Geometry: see drawing. Coordinates: mm, zero at the bounding-box minimum. Give positions to 0.01 mm unless a question says otherwise; leave off trailing zeros. Answer as a JSON object with one key per item and string values. Group by question number.
1. Material intervals for L1, parallel to Y at x = 3.25, z = 4.5 (1 decimal); L2, parallel to Y at x = 2.25, z = 10.75 (1 decimal); L3, parallel to Y at x = 5.75, z = 6.5, sorted ascending. Write a range as [from, to].
2. Section query A-A (x = 4). Count the separate pieces of the cut face and the enclosed holes in it, plus the area to 3 significant figures.
3. Pin query (flat end, axial travel): P1, Ø2, axis at x = 3.18, y = 52.39, coming from the +Z side. Return the tip coordinate at first contact, or that it passes through.
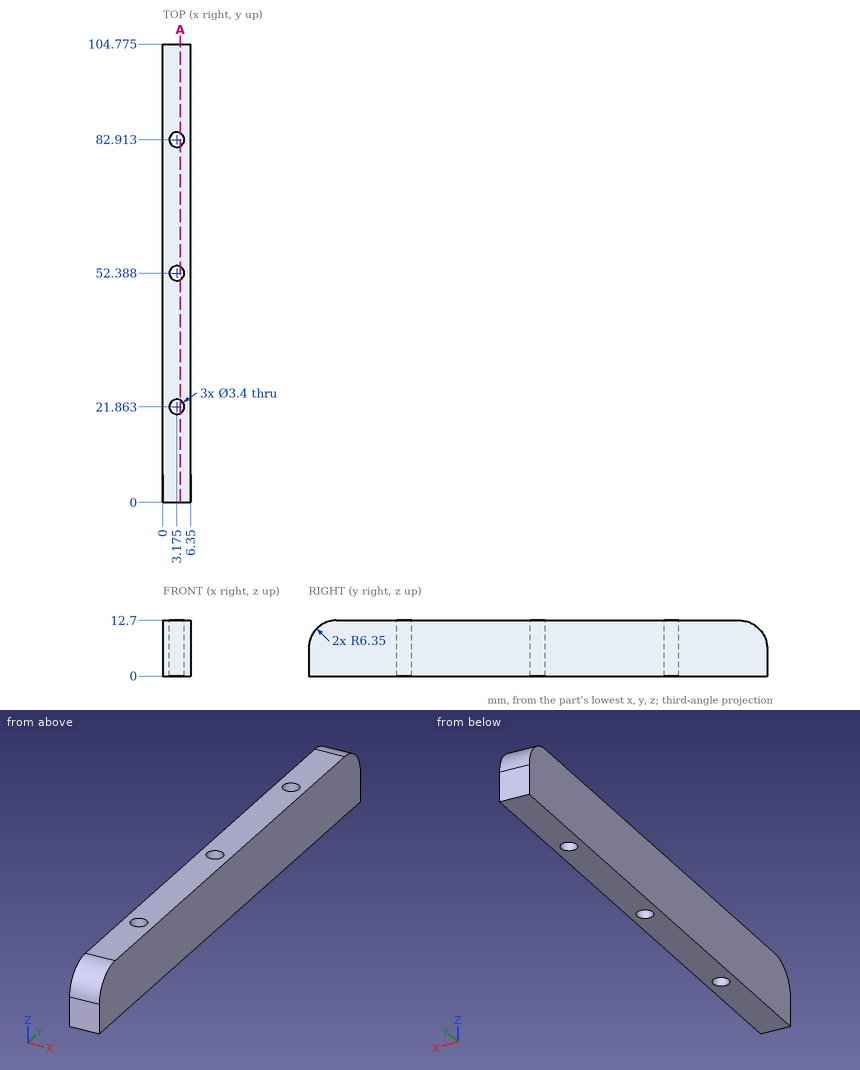
Answer sheet:
{
 "1": {"L1": "[0, 20.2], [23.6, 50.7], [54.1, 81.2], [84.6, 104.8]", "L2": "[1.8, 20.4], [23.3, 51], [53.8, 81.5], [84.3, 103]", "L3": "[0, 104.77]"},
 "2": {"separate pieces": "4", "enclosed holes": "0", "area": "1,200 mm^2"},
 "3": {"P1": "through"}
}
